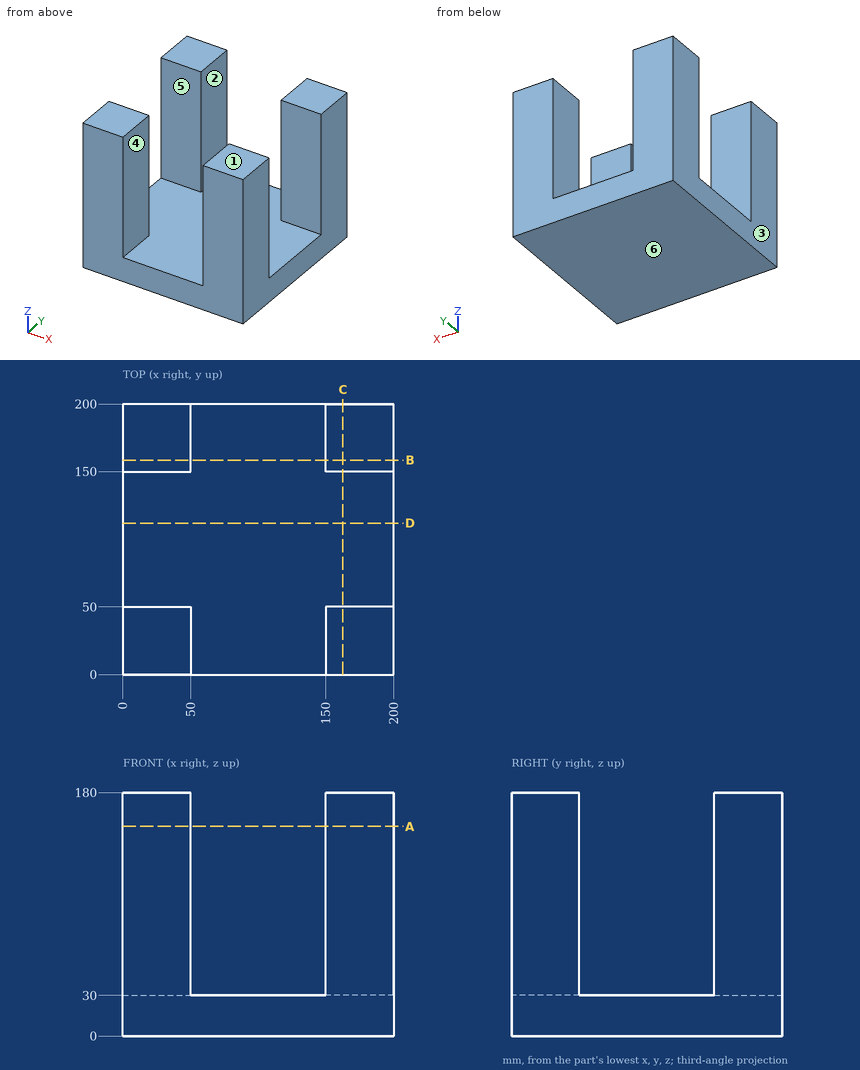
The drawing under review shows one solid part. Ordinate dimensions are in mm from its lowest x, y, z. A direction names the side the tool comes from. Coordinates: 2 decimals unless noted, no trailing zeros. Order: outer loops, then holes, each group sorted by start corner. A loop starts at its lowest first (then second) coordinate and runs counter-clockwise, first axis right, second up. Notation, with made-up numbers: (55.25, 66) -> (93.25, 66) arc R13 cw to (93.25, 87) -> close; hole circle Ø5 at (-17.5, 19.5). An arc over 180 degrees is marked (long way). Use CSV: the item, a comma, the result in double quotes. Start each with the question number.
Item 1: We need section D-D, the plane y = 112. Give the boundary of the cut face in (x, z).
Item 2: Insertion check: pin 1 (12 mm diameter, centred on x = 167.5, y = 93.5, fed in from +Z). The pin has a flat end and moves straight along its axis. Give the tip position at first contact, or say it passes through.
Item 3: Wall thickness on probe 1 along Y at (x, z) = (157, 82.5); probe 2 along Z at (x, y) = (70.5, 122.5): over which ranges is each line inside the solid? List them lowest first.
Item 4: We need section A-A, the plane z = 155. Give the boundary of the cut face in (x, y).
Item 5: Draft analysis for pull direction X (two halves, no side actions). For the marked faces 1, 2 and 3, state which applies: pulls with the +X half, pulls with the -X half, needs draft (parallel to the pull), parting line crosses it, or undercut.
Item 6: We need section B-B, the plane y = 158.5. Give the boundary of the cut face in (x, z), then the cut area to 3 significant figures.
Item 7: For the marked faces 4, 5 and 6, list the 3-axis set-ups (+Z, -Z, +X, -X, +Y, -Y) from which the entire face can be reached by the end or side of a thin tool; tool diameter is ignored.
Derived:
1,outline,"(0, 0) -> (200, 0) -> (200, 30) -> (0, 30) -> close"
2,pin 1,"stops at z = 30"
3,probe 1,"y = 0 to 50, 150 to 200"
3,probe 2,"z = 0 to 30"
4,outline,"(0, 0) -> (50, 0) -> (50, 50) -> (0, 50) -> close; (0, 150) -> (50, 150) -> (50, 200) -> (0, 200) -> close; (150, 0) -> (200, 0) -> (200, 50) -> (150, 50) -> close; (150, 150) -> (200, 150) -> (200, 200) -> (150, 200) -> close"
5,face 1,"needs draft"
5,face 2,"undercut"
5,face 3,"pulls with the -X half"
6,outline,"(0, 0) -> (200, 0) -> (200, 180) -> (150, 180) -> (150, 30) -> (50, 30) -> (50, 180) -> (0, 180) -> close"
6,area,"21,000 mm^2"
7,face 4,"+Z, +Y, -Y"
7,face 5,"+Z, +X, -X"
7,face 6,"-Z, +X, -X, +Y, -Y"
